Could you check a few things on this model? Use its own coordinates, in mm. Face numbers are marked on the shaded views. A direction names the side the tool comes from. Round coordinates to 2 decimals unless told otherwise and drop trailing zeros. Loops run counter-clockwise (first coordinate to the right, second up) from the corner with the lowest first, then second, coordinate; pieces in that order, holes last.
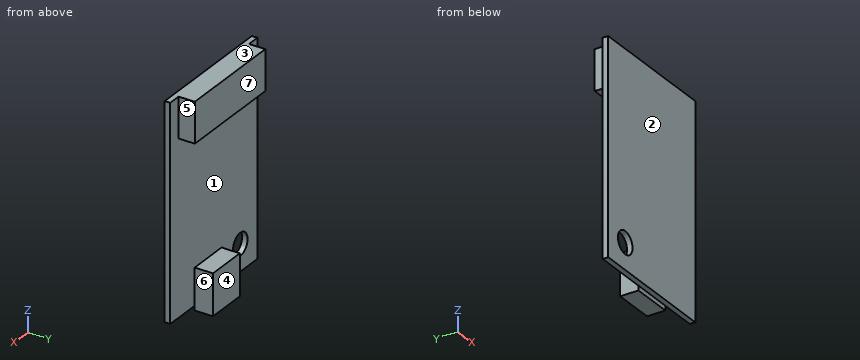
from build123d import *

# Parameters (mm, degrees)
SKETCH1_W           = 14.605
SKETCH1_H           = 23.1775
BOSS_EXTRUDE1_DEPTH = 0.6
SKETCH2_R           = 1.2192
CUT_EXTRUDE1_DEPTH  = 14.710785273
SKETCH3_W           = 11.811
SKETCH3_H           = 4.3942
BOSS_EXTRUDE2_DEPTH = 1.778
SKETCH4_W           = 4.5
SKETCH4_H           = 4.5
BOSS_EXTRUDE3_DEPTH = 2


with BuildPart() as part:
    # Sketch1 → Boss-Extrude1 (new body)
    with BuildSketch(Plane(origin=(0, 0, 0), x_dir=(1, 0, 0), z_dir=(0, 1, 0))):
        Rectangle(SKETCH1_W, SKETCH1_H)
    extrude(amount=BOSS_EXTRUDE1_DEPTH)

    # Sketch2 → Cut-Extrude1 (cut, through all)
    with BuildSketch(Plane(origin=(0, 0.6, 0), x_dir=(1, 0, 0), z_dir=(0, 1, 0))):
        with Locations(Location((-4.445, 8.73125, 0), (0, 0, 270))):
            Circle(SKETCH2_R)
    extrude(amount=-CUT_EXTRUDE1_DEPTH, mode=Mode.SUBTRACT)

    # Sketch3 → Boss-Extrude2 (add)
    with BuildSketch(Plane(origin=(0, 0.6, 0.6), x_dir=(1, 0, 0), z_dir=(0, 1, 0))):
        with Locations((0, -8.79165)):
            Rectangle(SKETCH3_W, SKETCH3_H)
    extrude(amount=BOSS_EXTRUDE2_DEPTH)

    # Sketch4 → Boss-Extrude3 (add)
    with BuildSketch(Plane(origin=(0, 0.6, 0), x_dir=(1, 0, 0), z_dir=(0, 1, 0))):
        with Locations((0.9525, 9.83875)):
            Rectangle(SKETCH4_W, SKETCH4_H)
    extrude(amount=BOSS_EXTRUDE3_DEPTH)


solid = part.part
Item 1: If we section it at A-A, the plane y = 1.9: Please give me the cut outline in (x, z).
Results list:
outline: (-5.91, 7.19) - (5.91, 7.19) - (5.91, 11.59) - (-5.91, 11.59) - close; (-1.3, -12.09) - (3.2, -12.09) - (3.2, -7.59) - (-1.3, -7.59) - close
Item 2: If we section it at D-D, the plane x = -5: Please give me the cut outline in (y, z).
Results list:
outline: (0, -11.59) - (0.6, -11.59) - (0.6, -9.82) - (0, -9.82) - close; (0, -7.65) - (0.6, -7.65) - (0.6, 7.19) - (2.38, 7.19) - (2.38, 11.59) - (0, 11.59) - close
Item 3: If we section it at C-C, the plane z = 9.25: Please give me the cut outline in (x, y).
Results list:
outline: (-7.3, 0) - (7.3, 0) - (7.3, 0.6) - (5.91, 0.6) - (5.91, 2.38) - (-5.91, 2.38) - (-5.91, 0.6) - (-7.3, 0.6) - close
Item 4: If I drill on line 1 along Z through (x, y) = (1.75, 2.15); line 2 along Z through (x, y) = (3.5, 0.95); line 3 along Y through (x, z) = (5.5, 9.75), over which ranges is the centre line in solid material (lowest first)?
Results list:
line 1: z = -12.09 to -7.59, 7.19 to 11.59
line 2: z = 7.19 to 11.59
line 3: y = 0 to 2.38
Item 5: Will these pins go through, and if not, where does the flat tip stop? pin 1 (0.6 mm diameter, centred on y = 1, z = -10, fed in from +X); pin 2 (1.3 mm diameter, centred on x = -0.5, z = 10.5, fed in from +Y); pin 3 (2 mm diameter, centred on x = 0.5, z = -4, fed in from +Y).
Results list:
pin 1: stops at x = 3.2
pin 2: stops at y = 2.38
pin 3: stops at y = 0.6
Item 6: If we section it at B-B, the plane x = 2.25: Please give me the cut outline in (y, z).
Results list:
outline: (0, -11.59) - (0.6, -11.59) - (0.6, -12.09) - (2.6, -12.09) - (2.6, -7.59) - (0.6, -7.59) - (0.6, 7.19) - (2.38, 7.19) - (2.38, 11.59) - (0, 11.59) - close
Item 7: For the marked faces 4, 5, 6 and 7, which set-ups out of +Z, -Z, +X, -X, +Y, -Y let a thin tool reach every point of the face, with its end or its side?
Results list:
face 4: +Z, -Z, +X, -X, +Y
face 5: +Z, -Z, +X, +Y
face 6: -Z, +X, +Y
face 7: +Z, +X, -X, +Y
Item 8: We'd pull the mould along Z, two halves only. Please class the marked faces 1, 2 and 3: released by +Z, released by -Z, zero draft, split by the parting line, or undercut.
Results list:
face 1: undercut
face 2: zero draft
face 3: released by +Z
